from build123d import *

# Parameters (mm, degrees)
BOSS_EXTRUDE1_DEPTH = 25.4
SHELL1_T            = -6.35
SKETCH2_R           = 3.98145
SKETCH2_R_2         = 3.1877
CUT_EXTRUDE1_DEPTH  = 59.965239742


with BuildPart() as part:
    # Sketch1 → Boss-Extrude1 (new body)
    with BuildSketch(Plane(origin=(0, 0, 0), x_dir=(1, 0, 0), z_dir=(0, 1, 0))):
        with BuildLine():
            Line((13.2334, 0), (26.921911775, 11.34881606))
            ThreePointArc((26.921911775, 11.34881606), (32.2834, 22.7584), (26.921911775, 34.16798394))
            Line((26.921911775, 34.16798394), (13.2334, 45.5168))
            Line((13.2334, 45.5168), (0, 45.5168))
            ThreePointArc((0, 45.5168), (-22.7584, 22.7584), (0, 0))
            Line((0, 0), (13.2334, 0))
        make_face()
    extrude(amount=BOSS_EXTRUDE1_DEPTH)

    # Shell1
    shell1_openings = [part.faces().sort_by_distance(p)[0] for p in [
        (3.880100933, 25.4, -22.7584),
    ]]
    offset(amount=SHELL1_T, openings=shell1_openings, kind=Kind.INTERSECTION)

    # Sketch2 → Cut-Extrude1 (cut, through all)
    with BuildSketch(Plane(origin=(0, 6.35, 0), x_dir=(1, 0, 0), z_dir=(0, 1, 0))):
        with Locations(Location((0, 22.7584, 0), (0, 0, 270))):
            Circle(SKETCH2_R)
        with Locations(Location((17.4625, 22.7584, 0), (0, 0, 270))):
            Circle(SKETCH2_R_2)
    extrude(amount=-CUT_EXTRUDE1_DEPTH, mode=Mode.SUBTRACT)


solid = part.part
Source: CAD feature listing. Evaluate the final solid. Frame: model axes, mm. A direction names the side the tool comes from. Coordinates: 2 decimals unless noted, no trailing zeros. Order: outer loops, then holes, each group sorted by start corner. A loop starts at its lowest first (then second) coordinate and runs counter-clockwise, first axis right, second up.
Item 1: Cut plane C-C (y = 5). Return loops of the section in (x, z).
Output values:
outline: (0, -45.52) - (13.23, -45.52) - (26.92, -34.17) arc R14.82 ccw to (26.92, -11.35) - (13.23, 0) - (0, 0) arc R22.76 ccw to start; hole circle Ø7.96 at (0, -22.76); hole circle Ø6.38 at (17.46, -22.76)
Item 2: Pull-direction query (X, two-part tool) for faces 1 (the face through (32.282, 12.522, -22.576)), 2 (the face through (7, 13, 0)), 3 (the face through (6, 16, -39.167)); classes: pulls with the +X half, pulls with the -X half, needs draft (parallel to the pull), parting line crosses it, or undercut.
Output values:
face 1: pulls with the +X half
face 2: needs draft
face 3: undercut
Item 3: Cut plane B-B (z = -7). Return loops of the section in (x, y).
Output values:
outline: (-16.42, 0) - (21.68, 0) - (21.68, 25.4) - (11.73, 25.4) - (11.73, 6.35) - (-4.57, 6.35) - (-4.57, 25.4) - (-16.42, 25.4) - close
Item 4: Cut plane D-D (x = 23.5). Return loops of the section in (y, z) (3 decimals).
Output values:
outline: (0, -37.005) - (25.4, -37.005) - (25.4, -28.7) - (6.35, -28.7) - (6.35, -16.817) - (25.4, -16.817) - (25.4, -8.512) - (0, -8.512) - close
Item 5: Set-up query: faces 4 (the face through (-1.52, 3.22, -19.08)), 5 (the face through (16.82, 15.74, -11.22)). Return all of +Z, -Z, +X, -X, +Y, -Y with unobstructed straight access to the full face (end or side cutting, diameter ignored); none if empty.
Output values:
face 4: +Y, -Y
face 5: +Y
Item 6: Cut plane A-A (y = 21.75). Return loops of the section in (x, z), plus the area to 3 significant figures.
Output values:
outline: (0, -45.52) - (13.23, -45.52) - (26.92, -34.17) arc R14.82 ccw to (26.92, -11.35) - (13.23, 0) - (0, 0) arc R22.76 ccw to start; hole (0, -39.17) - (10.94, -39.17) - (22.87, -29.28) arc R8.47 ccw to (22.87, -16.24) - (10.94, -6.35) - (0, -6.35) arc R16.41 ccw to start
area: 885 mm2
Item 7: First-contact query: P1, Ø1.5, axis at y = 9.5, z = -26, coming from the -X side; P2, Ø4, axis at x = 17.5, y = 14.5, coming from the -Z side; P3, Ø5, axis at x = -2, y = 3.5, coming from the +Z side; P4, Ø1, axis at x = -11.5, y = 19, coming from the -Z side. Flat tips, straight axial feed; report the tip coordinate or a pass-through.
Output values:
P1: stops at x = -22.62
P2: stops at z = -43.64
P3: stops at z = 0
P4: stops at z = -42.68
Item 8: Material intervals for line 1 (X direction, y = 5.5, z = -23); line 2 (Z direction, x = 4.5, y = 21.75); line 3 (Y direction, x = 16.5, z = -32.5), sorted ascending.
Output values:
line 1: x = -22.76 to -3.97, 3.97 to 14.28, 20.64 to 32.28
line 2: z = -45.52 to -39.17, -6.35 to 0
line 3: y = 0 to 6.35
